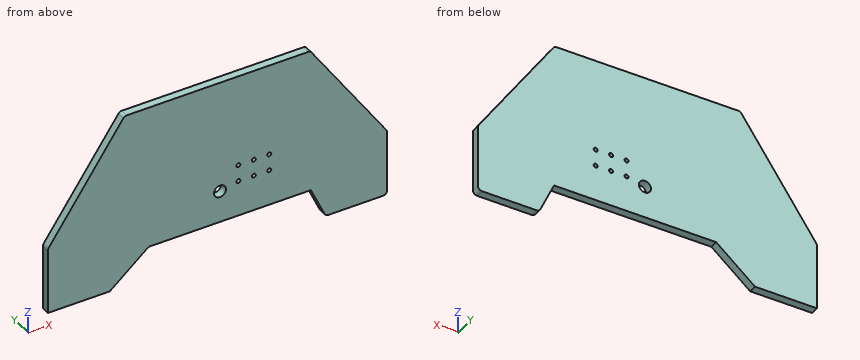
from build123d import *

# Parameters (mm, degrees)
BOSS_EXTRUDE1_DEPTH = 6.35
SKETCH2_R           = 3.175
CUT_EXTRUDE1_DEPTH  = 302.34078715
CUT_EXTRUDE2_DEPTH  = 302.34078715
FILLET1_R           = 6.35
SKETCH4_R           = 9.525
CUT_EXTRUDE3_DEPTH  = 302.34078715


with BuildPart() as part:
    # Sketch1 → Boss-Extrude1 (new, symmetric)
    with BuildSketch(Plane(origin=(0, 0, 0), x_dir=(1, 0, 0), z_dir=(0, 1, 0))):
        Polygon((-266.7, -139.7), (266.7, -139.7), (266.7, 139.7), (170.18, 139.7), (146.939, 88.9), (-108.237741638, 88.9), (-169.2275, 139.7), (-266.7, 139.7), align=None)
    extrude(amount=BOSS_EXTRUDE1_DEPTH, both=True)

    # Sketch2 → Cut-Extrude1 (cut, through all)
    with BuildSketch(Plane(origin=(0, 6.35, 0), x_dir=(1, 0, 0), z_dir=(0, 1, 0))):
        with Locations(Location((81.4832, 6.2484, 0), (0, 0, 270))):
            Circle(SKETCH2_R)
        with Locations(Location((81.4832, 32.4104, 0), (0, 0, 270))):
            Circle(SKETCH2_R)
        with Locations(Location((57.1627, 32.4104, 0), (0, 0, 270))):
            Circle(SKETCH2_R)
        with Locations(Location((32.8422, 32.4104, 0), (0, 0, 270))):
            Circle(SKETCH2_R)
        with Locations(Location((32.8422, 6.2484, 0), (0, 0, 270))):
            Circle(SKETCH2_R)
        with Locations(Location((57.1627, 6.2484, 0), (0, 0, 270))):
            Circle(SKETCH2_R)
    extrude(amount=-CUT_EXTRUDE1_DEPTH, mode=Mode.SUBTRACT)

    # Sketch3 → Cut-Extrude2 (cut, through all)
    with BuildSketch(Plane(origin=(0, 6.35, 0), x_dir=(1, 0, 0), z_dir=(0, 1, 0))):
        Polygon((-266.7, 34.925), (-146.05, -139.7), (-266.7, -139.7), align=None)
    cut_extrude2 = extrude(amount=-CUT_EXTRUDE2_DEPTH, mode=Mode.SUBTRACT)

    # Mirror1: Cut-Extrude2 across plane
    add(cut_extrude2.mirror(Plane(origin=(0, 0, 0), x_dir=(0, 0, 1), z_dir=(1, 0, 0))), mode=Mode.SUBTRACT)

    # Fillet1
    fillet1_edges = [part.edges().sort_by_distance(p)[0] for p in [
        (170.18, 0, -139.7),
        (266.7, 0, -139.7),
        (-266.7, 0, -34.925),
        (-146.05, 0, 139.7),
        (266.7, 0, -34.925),
        (146.05, 0, 139.7),
    ]]
    fillet(fillet1_edges, radius=FILLET1_R)

    # Sketch4 → Cut-Extrude3 (cut, through all)
    with BuildSketch(Plane(origin=(0, 6.35, 0), x_dir=(1, 0, 0), z_dir=(0, 1, 0))):
        with Locations(Location((3.99970692, 38.675446652, 0), (0, 0, 270))):
            Circle(SKETCH4_R)
    extrude(amount=-CUT_EXTRUDE3_DEPTH, mode=Mode.SUBTRACT)


solid = part.part
Part model, mm, in its own coordinate system. Give positions to 0.01 mm unless a question says otherwise; leave off trailing zeros. Order: outer loops, then holes, each group sorted by start corner. A loop starts at its lowest first (then second) coordinate and runs counter-clockwise, first axis right, second up. Notation, with made-up numbers: (-20.5, 42) - (-11.5, 42) arc R25 cw to (-11.5, 75) - close; hole circle Ø6 at (84, -12.5). An arc over 180 degrees is marked (long way). One line per question, with ' | ' between items.
1. Band-saw the part on C-C on x = -74. List the corners of the cut face in (y, z).
Filled in:
outline: (-6.35, -88.9) - (6.35, -88.9) - (6.35, 139.7) - (-6.35, 139.7) - close
2. Drop flat-ended pins along their axis: P1, Ø10, axis at x = 81.48, z = -6.25, coming from the +Y side; P2, Ø3, axis at x = -163, y = 1, coming from the +Z side; P3, Ø2, axis at x = -73, y = 3.5, coming from the -Z side; P4, Ø5.5, axis at x = 57.16, z = -32.41, coming from the +Y side. Give the stop position or say it passes through.
Filled in:
P1: y = 6.35 | P2: z = 117.34 | P3: z = -88.9 | P4: through
3. Band-saw the part on B-B on y = 1. Give the number of separate pieces and of enclosed holes in the cut face, then the cut area to 3 significant figures.
Filled in:
separate pieces: 1 | enclosed holes: 7 | area: 112,000 mm²
4. Band-saw the part on A-A on z = -117.5. List the corners of the cut face in (x, y).
Filled in:
outline: (-266.7, -6.35) - (-142.57, -6.35) - (-142.57, 6.35) - (-266.7, 6.35) - close; (160.02, -6.35) - (266.7, -6.35) - (266.7, 6.35) - (160.02, 6.35) - close
5. Band-saw the part on D-D on z = 25.5. List the corners of the cut face in (x, y), then the cut area to 3 significant figures.
Filled in:
outline: (-224.95, -6.35) - (224.95, -6.35) - (224.95, 6.35) - (-224.95, 6.35) - close | area: 5,710 mm²
6. Drill centre lines: probe 1 along Z at (x, y) = (138, -0.75); probe 2 along X at (y, z) = (-0.75, -102); probe 3 along Z at (x, y) = (-156, -4.5). Where is each one in solid material? Low to high.
Filled in:
probe 1: -88.9 to 139.7 | probe 2: -266.7 to -123.97, 152.93 to 266.7 | probe 3: -128.68 to 125.3
